Print and shaded views of the part. All mm, measured from the part's lowest x, y and z. A direction names the side the tool comes from. Coordinates: 2 decimals unless noted, no trailing zeros. Order: outer loops, then holes, each group sorted by start corner. A loop starts at its lowest first (then second) coordinate and runs counter-clockwise, first axis right, second up. Notation, with made-up numbers: (32, 41.5) - (82, 41.5) arc R21 cw to (82, 53.5) - close; hole circle Ø5 at (57, 15). An arc over 180 degrees is marked (long way). Write each question's results on one line, items separated by ' | '.
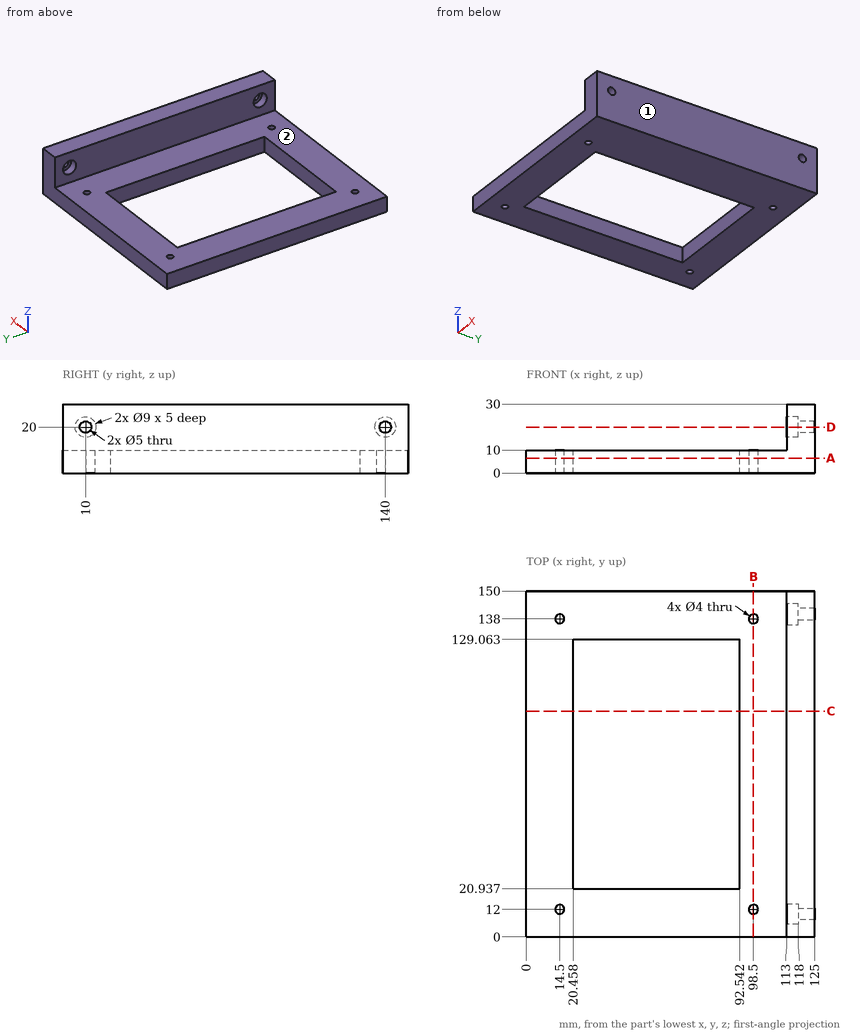
1. Band-saw the part on D-D on z = 20. Give the cut face in (x, y).
Solved:
outline: (113, 0) - (125, 0) - (125, 7.5) - (118, 7.5) - (118, 5.5) - (113, 5.5) - close; (113, 14.5) - (118, 14.5) - (118, 12.5) - (125, 12.5) - (125, 137.5) - (118, 137.5) - (118, 135.5) - (113, 135.5) - close; (113, 144.5) - (118, 144.5) - (118, 142.5) - (125, 142.5) - (125, 150) - (113, 150) - close
2. Tool access for the marked faces 1 and 2: list every direction of +Z, -Z, +X, -X, +Y, -Y with a clear straight run to the whole face (end or side of a thin tool).
Solved:
face 1: +Z, -Z, +X, +Y, -Y | face 2: +Z, -X, +Y, -Y
3. Band-saw the part on A-A on z = 6.5. Give the cut face in (x, y).
Solved:
outline: (0, 0) - (125, 0) - (125, 150) - (0, 150) - close; hole circle Ø4 at (14.5, 12); hole circle Ø4 at (14.5, 138); hole (20.46, 20.94) - (92.54, 20.94) - (92.54, 129.06) - (20.46, 129.06) - close; hole circle Ø4 at (98.5, 12); hole circle Ø4 at (98.5, 138)
4. Band-saw the part on C-C on y = 98. Give the cut face in (x, z).
Solved:
outline: (0, 0) - (20.46, 0) - (20.46, 10) - (0, 10) - close; (92.54, 0) - (125, 0) - (125, 30) - (113, 30) - (113, 10) - (92.54, 10) - close
5. Drop flat-ended pins along their axis: pin 1 Ø4 at (x, y) = (98.5, 61.5) entering from -Z; pin 2 Ø10 at (y, z) = (105.5, 23.5) entering from -X; pin 3 Ø4.5 at (y, z) = (9.5, 19) entering from -X; pin 4 Ø4.5 at (x, y) = (98.5, 12) entering from +Z. Give the stop position or say it passes through.
Solved:
pin 1: stops at z = 0 | pin 2: stops at x = 113 | pin 3: stops at x = 118 | pin 4: stops at z = 10
6. Probe line 1 (X direction, y = 138, z = 3.25); line 2 (Y direction, x = 98.5, z = 5); line 3 (Z direction, x = 119.5, y = 140). List the from-to ranges inside material, lowest first.
Solved:
line 1: x = 0 to 12.5, 16.5 to 96.5, 100.5 to 125 | line 2: y = 0 to 10, 14 to 136, 140 to 150 | line 3: z = 0 to 17.5, 22.5 to 30
7. Band-saw the part on B-B on x = 98.5. Give the cut face in (y, z).
Solved:
outline: (0, 0) - (10, 0) - (10, 10) - (0, 10) - close; (14, 0) - (136, 0) - (136, 10) - (14, 10) - close; (140, 0) - (150, 0) - (150, 10) - (140, 10) - close
